Input: part model. Units: mm. Frame: model coordinates. Face numbers are marked on the shaded views. Round coordinates to 2 decimals unless told otherwise and drop trailing zeros. Loops run counter-clockwise (first coordinate to the right, second up) from the corner with the lowest first, then second, coordinate; pieces in that order, holes last. Notation, with made-up numbers: (54.25, -11.5) -> (87.25, -11.5) arc R24 ccw to (87.25, 11.5) -> close; hole circle Ø2 at (-32.75, 20). An arc over 180 degrees is marked (long way). Answer in a Markdown table with one row per item. Add a question column.
Q1. Pin query (flat end, axial travel): pin 1 (1.5 mm diameter, centred on x = -2, z = -3, fed in from -Y); pin 2 (1 mm diameter, centred on x = -5, y = -22.5, fed in from +Z). Return the tip coordinate at first contact, or that it passes through.
Q2. Ray query, L1, parallel to X at y = -10.5, z = -1.25; L2, parallel to Z at x = -5, y = -20.25; L3, parallel to X at y = -9.5, z = -3.75. Return the intervals inside material, ascending. Write a range as from..to.
Q3. Section A-A, the plane z = -4.25. Output: boundary loops of the cut face in (x, y), and give its area (3 significant figures).
Q4. Section C-C, the plane y = -14. Output: boundary loops of the cut face in (x, z).
Q5. Section B-B, the plane x = 17. Output: boundary loops of the cut face in (y, z), and give its area (3 significant figures).
Q6. Mould query, pull axis X, two halves, no side actions, for the marked faces 1, 2, 3 and 4. Classes: pulls with the +X half, pulls with the -X half, needs draft (parallel to the pull), parting line crosses it, or undercut.
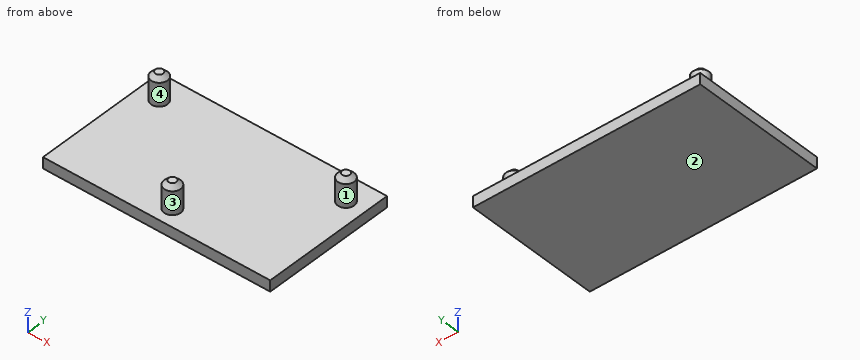
Autodesk Inventor part; units mm, degrees
ref_plane "YZ Plane" through (0, 0, 0) normal (1, 0, 0) x (0, 1, 0)
ref_plane "XZ Plane" through (0, 0, 0) normal (0, 1, 0) x (-1, 0, 0)
ref_plane "XY Plane" through (0, 0, 0) normal (0, 0, 1) x (1, 0, 0)
ref_plane "Work Plane3" through (6.1355, -21.1735, -7.3328) normal (0, 0, 1) x (1, 0, 0)
sketch "Sketch3" plane through (6.1355, -21.1735, -7.3328) normal (0, 0, 1) x (1, 0, 0)
  line L0 (20.5093, -9.3897) -> (-20.8066, -9.3897)
  line L1 (-20.8066, -9.3897) -> (-20.8066, 15.1082)
  line L2 (-20.8066, 15.1082) -> (20.5093, 15.1082)
  line L3 (20.5093, 15.1082) -> (20.5093, -9.3897)
  line L4 (-12.3, 2) -> (7, 2)
  circle A0 centre (16.975, 10.575) radius 1.621
  circle A1 centre (0, -6.25) radius 1.621
  circle A2 centre (-16.975, 10.575) radius 1.621
  line L5 (-19.5, 23) -> (-19.5, -23)
  line L6 (-19.5, -23) -> (-13.8, -23)
  line L7 (-13.8, -23) -> (-13.8, -17.4)
  arc A3 (-10.8, -14.4) -> (-13.8, -17.4) centre (-10.8, -17.4) ccw
  line L8 (-10.8, -14.4) -> (10.8, -14.4)
  arc A4 (13.8, -17.4) -> (10.8, -14.4) centre (10.8, -17.4) ccw
  line L9 (13.8, -17.4) -> (13.8, -23)
  line L10 (13.8, -23) -> (19.5, -23)
  line L11 (19.5, -23) -> (19.5, 23)
  line L12 (19.5, 23) -> (-19.5, 23)
  circle A5 centre (-17, -20) radius 1.25
  circle A6 centre (17, -20) radius 1.25
  circle A7 centre (17, 20) radius 1.25
  circle A8 centre (-17, 20) radius 1.25
  circle A9 centre (0, -6.25) radius 1.5
  circle A10 centre (16.975, 10.575) radius 1.5
  circle A11 centre (-16.975, 10.575) radius 1.5
  point P0 (-6.1355, 21.1735)
  dimension "d18" = 3
  dimension "d19" = 3
  dimension "d20" = 3
extrude "Extrusion3" add sketch "Sketch3" along normal blind 2 contours L0 L11 L2 L3 | L0 L5 L2 L11 | L0 L1 L2 L5 | A0 | A1 | A2 | A9 | A10 | A11
sketch "Sketch4" plane through (6.1355, -21.1735, -5.3328) normal (0, 0, 1) x (1, 0, 0)
  circle A0 centre (16.975, 10.575) radius 1.621
  circle A1 centre (0, -6.25) radius 1.621
  circle A2 centre (-16.975, 10.575) radius 1.621
  line L0 (-19.5, 23) -> (-19.5, -23)
  line L1 (-19.5, -23) -> (-13.8, -23)
  line L2 (-13.8, -23) -> (-13.8, -17.4)
  arc A3 (-10.8, -14.4) -> (-13.8, -17.4) centre (-10.8, -17.4) ccw
  line L3 (-10.8, -14.4) -> (10.8, -14.4)
  arc A4 (13.8, -17.4) -> (10.8, -14.4) centre (10.8, -17.4) ccw
  line L4 (13.8, -17.4) -> (13.8, -23)
  line L5 (13.8, -23) -> (19.5, -23)
  line L6 (19.5, -23) -> (19.5, 23)
  line L7 (19.5, 23) -> (-19.5, 23)
  circle A5 centre (-17, -20) radius 1.25
  circle A6 centre (17, -20) radius 1.25
  circle A7 centre (17, 20) radius 1.25
  circle A8 centre (-17, 20) radius 1.25
  circle A9 centre (0, -6.25) radius 1.5
  circle A10 centre (-16.975, 10.575) radius 1.5
  circle A11 centre (16.975, 10.575) radius 1.5
  point P0 (-6.1355, 21.1735)
  dimension "d23" = 3
  dimension "d24" = 3
  dimension "d25" = 3
extrude "Extrusion4" add sketch "Sketch4" along normal blind 5 contours A9 | A10 | A11
chamfer "Chamfer2" distance 0.8 angle 45 3 edges at (21.6105, -10.5985, -0.3328) (4.6355, -27.4235, -0.3328) (-12.3395, -10.5985, -0.3328)
properties part number "vesc_holes_check"
Answer block:
| question | item | result |
|---|---|---|
| 1 | pin 1 | through |
| 1 | pin 2 | z = -5.33 |
| 2 | L1 | -12.34..-9.34, 21.61..24.61 |
| 2 | L2 | -7.33..-5.33 |
| 2 | L3 | -11.86..-9.82, 22.09..24.13 |
| 3 | outline | circle Ø3 at (-10.84, -10.6); circle Ø3 at (6.14, -27.42); circle Ø3 at (23.11, -10.6) |
| 3 | area | 21.2 mm^2 |
| 4 | outline | (-14.67, -7.33) -> (26.64, -7.33) -> (26.64, -5.33) -> (-14.67, -5.33) -> close |
| 5 | outline | (-30.56, -7.33) -> (-6.07, -7.33) -> (-6.07, -5.33) -> (-30.56, -5.33) -> close |
| 5 | area | 49.0 mm^2 |
| 6 | face 1 | undercut |
| 6 | face 2 | needs draft |
| 6 | face 3 | parting line crosses it |
| 6 | face 4 | undercut |
